Source: CAD feature listing. Evaluate the final solid. Frame: model axes, mm. A direction names the side the tool comes from. Round coordinates to 2 decimals unless told otherwise and drop trailing zeros. Order: outer loops, then holes, each group sorted by start corner. A loop starts at its lowest first (then second) coordinate and runs counter-clockwise, first axis right, second up.
```python
from build123d import *

# Parameters (mm, degrees)
MAIN_STOCK_START                   = 2.248090434
SKETCH_1_W                         = 4
SKETCH_1_H                         = 46.98
MAIN_STOCK_DEPTH                   = 8.851909566
SKETCH_2_R                         = 0.8
FRAME_1XD1P6_THROUGH_DEPTH         = 70.124968014
SKETCH_3_R                         = 2.05
SMA_CENTER_D4P1_DEPTH              = 4
SKETCH_4_R                         = 0.875
SMA_UPPER_2XD1P75_THROUGH_DEPTH    = 45.280835584
SKETCH_5_W                         = 6.7
SKETCH_5_H                         = 11.5
TYPEC_WINDOW_11P5X6P7_DEPTH        = 4
SKETCH_6_R                         = 1.1
CORNER_FRONT_2XD2P2_THROUGH_DEPTH  = 45.280835584
SKETCH_7_R                         = 0.8
CORNER_REAR_2XD1P6_BLIND4_DEPTH    = 4
SKETCH_8_W                         = 4
SKETCH_8_H                         = 46.98
WALL_EXTENSION_TO_FLOOR_DEPTH      = 5
SKETCH_9_R                         = 2.05
SMA_CENTER_FULL_BORE_DEPTH         = 4.01
SKETCH_10_R                        = 0.875
SMA_LOWER_M2P2_THROUGH_DEPTH       = 4.01
SKETCH_11_W                        = 6.7
SKETCH_11_H                        = 11.5
RIGHT_WINDOW_FULL_11P5X6P7_DEPTH   = 4.01
SKETCH_12_R                        = 1.1
HORIZONTAL_BASE_M2_0_0_05365_DEPTH = 4.01


with BuildPart() as part:
    # 草图1 → Main_Stock (new body)
    with BuildSketch(Plane.XY.offset(MAIN_STOCK_START)):
        with Locations((51.65, 19.19)):
            Rectangle(SKETCH_1_W, SKETCH_1_H)
    extrude(amount=MAIN_STOCK_DEPTH)

    # 草图2 → Frame_1xD1p6_Through (cut, through all)
    with BuildSketch(Plane.XY.offset(11.1)):
        with Locations((51.65, 1)):
            Circle(SKETCH_2_R)
    extrude(amount=-FRAME_1XD1P6_THROUGH_DEPTH, mode=Mode.SUBTRACT)

    # 草图3 → SMA_Center_D4p1 (cut)
    with BuildSketch(Plane(origin=(53.65, 0, 0), x_dir=(0, 0, -1), z_dir=(1, 0, 0))):
        with Locations((-3.899496327, 10.725)):
            Circle(SKETCH_3_R)
    extrude(amount=-SMA_CENTER_D4P1_DEPTH, mode=Mode.SUBTRACT)

    # 草图4 → SMA_Upper_2xD1p75_Through (cut, through all)
    with BuildSketch(Plane(origin=(53.65, 0, 0), x_dir=(0, 0, -1), z_dir=(1, 0, 0))):
        with Locations((-8.199496327, 6.425)):
            Circle(SKETCH_4_R)
        with Locations((-8.199496327, 15.025)):
            Circle(SKETCH_4_R)
    extrude(amount=-SMA_UPPER_2XD1P75_THROUGH_DEPTH, mode=Mode.SUBTRACT)

    # 草图5 → TypeC_Window_11p5x6p7 (cut)
    with BuildSketch(Plane(origin=(53.65, 0, 0), x_dir=(0, 0, -1), z_dir=(1, 0, 0))):
        with Locations((-4.25, 31.65)):
            Rectangle(SKETCH_5_W, SKETCH_5_H)
    extrude(amount=-TYPEC_WINDOW_11P5X6P7_DEPTH, mode=Mode.SUBTRACT)

    # 草图6 → Corner_Front_2xD2p2_Through (cut, through all)
    with BuildSketch(Plane(origin=(53.65, 0, 0), x_dir=(0, 0, -1), z_dir=(1, 0, 0))):
        with Locations((-5.1, -2.3)):
            Circle(SKETCH_6_R)
        with Locations((-9.1, -2.3)):
            Circle(SKETCH_6_R)
    extrude(amount=-CORNER_FRONT_2XD2P2_THROUGH_DEPTH, mode=Mode.SUBTRACT)

    # 草图7 → Corner_Rear_2xD1p6_Blind4 (cut)
    with BuildSketch(Plane(origin=(0, 42.68, 0), x_dir=(1, 0, 0), z_dir=(0, 1, 0))):
        with Locations(Location((51.65, -5.1, 0), (0, 0, 270))):
            Circle(SKETCH_7_R)
        with Locations(Location((51.65, -9.1, 0), (0, 0, 270))):
            Circle(SKETCH_7_R)
    extrude(amount=-CORNER_REAR_2XD1P6_BLIND4_DEPTH, mode=Mode.SUBTRACT)

    # 草图8 → Wall_Extension_To_Floor (add)
    with BuildSketch(Plane(origin=(0, 0, 2.248090434), x_dir=(-1, 0, 0), z_dir=(0, 0, -1))):
        with Locations((-51.65, 19.19)):
            Rectangle(SKETCH_8_W, SKETCH_8_H)
    extrude(amount=WALL_EXTENSION_TO_FLOOR_DEPTH)

    # 草图9 → SMA_Center_Full_Bore (cut)
    with BuildSketch(Plane(origin=(53.65, 0, 0), x_dir=(0, 0, -1), z_dir=(1, 0, 0))):
        with Locations((-3.899496327, 10.725)):
            Circle(SKETCH_9_R)
    extrude(amount=-SMA_CENTER_FULL_BORE_DEPTH, mode=Mode.SUBTRACT)

    # 草图10 → SMA_Lower_M2p2_Through (cut)
    with BuildSketch(Plane(origin=(53.65, 0, 0), x_dir=(0, 0, -1), z_dir=(1, 0, 0))):
        with Locations((0.400503673, 6.425)):
            Circle(SKETCH_10_R)
        with Locations((0.400503673, 15.025)):
            Circle(SKETCH_10_R)
    extrude(amount=-SMA_LOWER_M2P2_THROUGH_DEPTH, mode=Mode.SUBTRACT)

    # 草图11 → Right_Window_Full_11p5x6p7 (cut)
    with BuildSketch(Plane(origin=(53.65, 0, 0), x_dir=(0, 0, -1), z_dir=(1, 0, 0))):
        with Locations((-4.25, 31.65)):
            Rectangle(SKETCH_11_W, SKETCH_11_H)
    extrude(amount=-RIGHT_WINDOW_FULL_11P5X6P7_DEPTH, mode=Mode.SUBTRACT)

    # 草图12 → Horizontal_Base_M2_0_0.05365 (cut)
    with BuildSketch(Plane(origin=(53.65, 0, 0), x_dir=(0, 0, -1), z_dir=(1, 0, 0))):
        with Locations((0.75, 20)):
            Circle(SKETCH_12_R)
        with Locations((0.75, 24)):
            Circle(SKETCH_12_R)
    extrude(amount=-HORIZONTAL_BASE_M2_0_0_05365_DEPTH, mode=Mode.SUBTRACT)


solid = part.part
```
1. Section B-B on y = -2.3. Return loops of the section in (x, z).
2. Access query for faces 1 (the face through (52, 38.68, 5)), 2 (the face through (52, 1, 2.248)), 3 (the face through (52, 25.9, 4)), 4 (the face through (52, -4.3, 4)). Directions: +Z, -Z, +X, -X, +Y, -Y. A direction counts if a zero-diameter tool reaches every point of the face in a straight line with its end or side. Return the directions, or none.
3. Section D-D on z = 5.1. Return loops of the section in (x, y).
4. Section A-A on y = 24. Return loops of the section in (x, z), plus the area to 3 significant figures.
5. Pull-direction query (Z, two-part tool) for faces 5 (the face through (52, 20, 11.1)), 6 (the face through (51.678, 22.926, -0.512)), 7 (the face through (53.65, 19, 4)), 8 (the face through (52.325, 40.708, 5.53)); classes: released by +Z, released by -Z, zero draft, split by the parting line, or undercut.
6. Section C-C on z = -0.75. Return loops of the section in (x, y).
7. First-contact query: pin 1 (0.8 mm diameter, centred on x = 51.5, z = 5, fed in from +Y). Flat tip, straight axial feed; report the tip coordinate or a pass-through.
8. Line query: line 1 along Z through (x, y) = (51.65, 40.95); line 2 along Y through (x, z) = (50.45, 1.25); line 3 along Y through (x, z) = (50.6, 2.75). Output: solid intervals per line, ascending.
Result:
1. outline: (49.65, -2.75) - (53.65, -2.75) - (53.65, 4) - (49.65, 4) - close; (49.65, 6.2) - (53.65, 6.2) - (53.65, 8) - (49.65, 8) - close; (49.65, 10.2) - (53.65, 10.2) - (53.65, 11.1) - (49.65, 11.1) - close
2. face 1: +Y
2. face 2: +Z
2. face 3: +X, -X
2. face 4: +Z, -Z, +X, -X, -Y
3. outline: (49.65, -4.3) - (53.65, -4.3) - (53.65, -3.4) - (49.65, -3.4) - close; (49.65, -1.2) - (53.65, -1.2) - (53.65, 9.06) - (49.65, 9.06) - close; (49.65, 12.39) - (53.65, 12.39) - (53.65, 25.9) - (49.65, 25.9) - close; (49.65, 37.4) - (53.65, 37.4) - (53.65, 42.68) - (52.45, 42.68) - (52.45, 38.68) - (50.85, 38.68) - (50.85, 42.68) - (49.65, 42.68) - close; hole circle Ø1.6 at (51.65, 1)
4. outline: (49.65, -2.75) - (53.65, -2.75) - (53.65, -1.85) - (49.65, -1.85) - close; (49.65, 0.35) - (53.65, 0.35) - (53.65, 11.1) - (49.65, 11.1) - close
4. area: 46.6 mm2
5. face 5: released by +Z
5. face 6: undercut
5. face 7: zero draft
5. face 8: undercut
6. outline: (49.65, -4.3) - (53.65, -4.3) - (53.65, 5.62) - (49.65, 5.62) - close; (49.65, 7.23) - (53.65, 7.23) - (53.65, 14.22) - (49.65, 14.22) - close; (49.65, 15.83) - (53.65, 15.83) - (53.65, 18.9) - (49.65, 18.9) - close; (49.65, 21.1) - (53.65, 21.1) - (53.65, 22.9) - (49.65, 22.9) - close; (49.65, 25.1) - (53.65, 25.1) - (53.65, 42.68) - (49.65, 42.68) - close
7. pin 1: stops at y = 38.68
8. line 1: z = -2.75 to 4.3, 5.9 to 8.3, 9.9 to 11.1
8. line 2: y = -4.3 to 25.9, 37.4 to 42.68
8. line 3: y = -4.3 to 9.03, 12.42 to 25.9, 37.4 to 42.68
